Work out the finished part from the listing and answer in its coordinate system (mm). A direction names the side the tool comes from. Give positions to 0.01 mm unless a question says otherwise; leave off trailing zeros. Order: outer loops, then holes, each group sorted by start corner. A loop starts at its lowest first (then second) coordinate and runs counter-clockwise, first axis right, second up. Notation, with made-up numbers: (-15.75, 89) - (30.25, 89) arc R13 ccw to (30.25, 95) - close; hole circle Ø1 at (82.25, -14.75). An arc over 180 degrees is marked (long way). Put each result on its own line as item: value.
```python
from build123d import *

# Parameters (mm, degrees)
SKETCH1_R           = 23.5
SKETCH1_R_2         = 17.5
BOSS_EXTRUDE1_DEPTH = 7
SKETCH2_R           = 22
SKETCH2_R_2         = 19
CUT_EXTRUDE1_DEPTH  = 0.2
CHAMFER1_SIZE       = 0.3
SKETCH3_R           = 22
SKETCH3_R_2         = 19
CUT_EXTRUDE2_DEPTH  = 0.2


with BuildPart() as part:
    # Sketch1 → Boss-Extrude1 (new body)
    with BuildSketch(Plane(origin=(0, 0, 0), x_dir=(1, 0, 0), z_dir=(0, 1, 0))):
        Circle(SKETCH1_R)
        Circle(SKETCH1_R_2, mode=Mode.SUBTRACT)
    extrude(amount=BOSS_EXTRUDE1_DEPTH)

    # Sketch2 → Cut-Extrude1 (cut)
    with BuildSketch(Plane(origin=(0, 7, 0), x_dir=(1, 0, 0), z_dir=(0, 1, 0))):
        Circle(SKETCH2_R)
        Circle(SKETCH2_R_2, mode=Mode.SUBTRACT)
    extrude(amount=-CUT_EXTRUDE1_DEPTH, mode=Mode.SUBTRACT)

    # Chamfer1
    chamfer1_edges = [part.edges().sort_by_distance(p)[0] for p in [
        (-23.5, 0, 0),
        (-23.5, 7, 0),
        (-17.5, 0, 0),
        (-17.5, 7, 0),
    ]]
    chamfer(chamfer1_edges, length=CHAMFER1_SIZE)

    # Sketch3 → Cut-Extrude2 (cut)
    with BuildSketch(Plane.XZ):
        Circle(SKETCH3_R)
        Circle(SKETCH3_R_2, mode=Mode.SUBTRACT)
    extrude(amount=-CUT_EXTRUDE2_DEPTH, mode=Mode.SUBTRACT)


solid = part.part
```
(1) Given pin 1 (1 mm diameter, centred on x = 12, y = 4, fed in from +Z); pin 2 (2 mm diameter, centred on x = 13, y = 1, fed in from -Z); pin 3 (3 mm diameter, centred on x = -15, z = 0, fed in from -Y); pin 4 (1.5 mm diameter, centred on y = 2.5, z = -3.5, fed in from -X), each flat-ended and moving along its own axis, determine where each tip first touches the part or whether it passes through.
Geometry check:
pin 1: stops at z = 20.49
pin 2: stops at z = -20.21
pin 3: passes through
pin 4: stops at x = -23.34
(2) A tool of negligible diameter and unlimited length cuts with its end or side. For faces 5 (the face through (-17, 7, 6)), 6 (the face through (-7, 6.8, -18)), from which of +Z, -Z, +X, -X, +Y, -Y can it reach the whole face along a straight path? Write none if from no direction.
Geometry check:
face 5: +Z, -Z, +X, -X, +Y
face 6: +Y
(3) Section C-C, the plane y = 3 is taken. Write down the section's boundary in (x, z), then the cut area to 3 significant figures.
Geometry check:
outline: circle Ø47 at (0, 0); hole circle Ø35 at (0, 0)
area: 773 mm²
(4) Determine the mould class of faces 1 (the face through (-7, 0.2, 18)), 2 (the face through (-13.887, 3.455, 10.648)), 3 (the face through (8, 0, 21)), 4 (the face through (22.4, 3.5, -7.1)) for opening direction X: pulls with the +X half, pulls with the -X half, needs draft (parallel to the pull), parting line crosses it, or undercut.
Geometry check:
face 1: undercut
face 2: undercut
face 3: needs draft
face 4: parting line crosses it
(5) Straight lines are drawn through the part: line 1 (Z direction, x = 0, y = 3.25); line 2 (X direction, y = 6.9, z = 0). For each, find the intervals that lie inside material, in ascending order.
Geometry check:
line 1: z = -23.5 to -17.5, 17.5 to 23.5
line 2: x = -23.3 to -22, -19 to -17.7, 17.7 to 19, 22 to 23.3
